```python
from build123d import *

# Parameters (mm, degrees)
BOSS_EXTRUDE1_DEPTH = 0.8
BOSS_EXTRUDE2_DEPTH = 1
BOSS_EXTRUDE3_START = 1
BOSS_EXTRUDE3_DEPTH = 1
CUT_EXTRUDE1_DEPTH  = 0.5
SKETCH5_W           = 18.969303985
SKETCH5_H           = 16.990491699
CUT_EXTRUDE2_DEPTH  = 4


with BuildPart() as part:
    # Sketch1 → Boss-Extrude1 (new body)
    with BuildSketch(Plane(origin=(0, 0, 0), x_dir=(1, 0, 0), z_dir=(0, 1, 0))):
        with BuildLine():
            Line((-5, 7.5), (-5, 5.590169944))
            ThreePointArc((-5, 5.590169944), (-6.846531969, 3.061862178), (-7.5, 0))
            Line((-7.5, 0), (-7.5, -7.5))
            Line((-7.5, -7.5), (7.5, -7.5))
            Line((7.5, -7.5), (7.5, 0))
            ThreePointArc((7.5, 0), (6.846531969, 3.061862178), (5, 5.590169944))
            Line((5, 5.590169944), (5, 7.5))
            Line((5, 7.5), (3, 7.5))
            Line((3, 7.5), (3, 5.5))
            Line((3, 5.5), (3, 5.123475383))
            ThreePointArc((3, 5.123475383), (3.101282966, 4.684946373), (3.384615385, 4.335248401))
            ThreePointArc((3.384615385, 4.335248401), (0, -5.5), (-3.384615385, 4.335248401))
            ThreePointArc((-3.384615385, 4.335248401), (-3.101282966, 4.684946373), (-3, 5.123475383))
            Line((-3, 5.123475383), (-3, 5.5))
            Line((-3, 5.5), (-3, 7.5))
            Line((-3, 7.5), (-5, 7.5))
        make_face()
    extrude(amount=BOSS_EXTRUDE1_DEPTH)

    # Sketch2 → Boss-Extrude2 (add)
    with BuildSketch(Plane(origin=(0, 0.8, 0), x_dir=(1, 0, 0), z_dir=(0, 1, 0))):
        with BuildLine():
            Line((5, 5.590169944), (5, 7.5))
            Line((5, 7.5), (3, 7.5))
            Line((3, 7.5), (-3, 7.5))
            Line((-3, 7.5), (-5, 7.5))
            Line((-5, 7.5), (-5, 5.590169944))
            ThreePointArc((-5, 5.590169944), (-6.846531969, 3.061862178), (-7.5, 0))
            Line((-7.5, 0), (-7.5, -7.5))
            Line((-7.5, -7.5), (7.5, -7.5))
            Line((7.5, -7.5), (7.5, 0))
            ThreePointArc((7.5, 0), (6.846531969, 3.061862178), (5, 5.590169944))
        make_face()
    extrude(amount=BOSS_EXTRUDE2_DEPTH)

    # Sketch3 → Boss-Extrude3 (add)
    with BuildSketch(Plane.XZ.offset(BOSS_EXTRUDE3_START)):
        with BuildLine():
            Line((-3, -7.5), (-5, -7.5))
            Line((-5, -7.5), (-5, -5.590169944))
            ThreePointArc((-5, -5.590169944), (-6.846531969, -3.061862178), (-7.5, 0))
            Line((-7.5, 0), (-7.5, 7.5))
            Line((-7.5, 7.5), (7.5, 7.5))
            Line((7.5, 7.5), (7.5, 0))
            ThreePointArc((7.5, 0), (6.846531969, -3.061862178), (5, -5.590169944))
            Line((5, -5.590169944), (5, -7.5))
            Line((5, -7.5), (3, -7.5))
            Line((3, -7.5), (-3, -7.5))
        make_face()
    extrude(amount=-BOSS_EXTRUDE3_DEPTH)

    # Sketch4 → Cut-Extrude1 (cut)
    with BuildSketch(Plane(origin=(0, 0, -7.5), x_dir=(-1, 0, 0), z_dir=(0, 0, -1))):
        Polygon((-5, 0.55), (-0.15, 0.55), (-0.15, 1.8), (0.15, 1.8), (0.15, 0.55), (5, 0.55), (5, 0.25), (0.15, 0.25), (0.15, -1), (-0.15, -1), (-0.15, 0.25), (-5, 0.25), align=None)
    extrude(amount=-CUT_EXTRUDE1_DEPTH, mode=Mode.SUBTRACT)

    # Sketch5 → Cut-Extrude2 (cut)
    with BuildSketch(Plane(origin=(0, 0.4, 0), x_dir=(-1, 0, 0), z_dir=(0, -1, 0))):
        with Locations((0.318429563, 0.045489938)):
            Rectangle(SKETCH5_W, SKETCH5_H)
    extrude(amount=CUT_EXTRUDE2_DEPTH, mode=Mode.SUBTRACT)


solid = part.part
```
Can you work these out from the model? Positions are in its coordinate system, mm. A direction names the side the tool comes from. Give positions to 0.01 mm unless a question says otherwise; leave off trailing zeros. Loops run counter-clockwise (first coordinate to the right, second up) from the corner with the lowest first, then second, coordinate; pieces in that order, holes last. Notation, with made-up numbers: M -19,14.25 L 38,14.25 A25 cw 38,39.25 Z; hole C 14.25,6 d8. An arc over 180 degrees is marked long. Use one line per item in the form item = value. Start each with the question number.
(1) Thinking about a two-plate mould opening in Z: for faces 4 (the cylindrical face through (0.191, 0.597, 5.497)), 5 (the flat face through (-7.5, 1, 4)), 6 (the flat face through (-3, 1, -7.5)), which applies, released by +Z, released by -Z, zero draft, split by the parting line, or undercut?
(2) On a 3-axis mill with a long thin cutter (end or side, diameter ignored), from which of +Z, -Z, +X, -X, +Y, -Y can I reach the whole of each face in a straight line? I mean faces 1 (the flat face through (5, 1, -7)), 2 (the flat face through (0, 0.8, -1)), 3 (the flat face through (-5, 1, -7)). Say none if no direction works.
(3) Please list where these lines run through material, in increasing order: line 1 (X direction, y = 0.7, z = 0); line 2 (X direction, y = 0.5, z = -6); line 3 (Z direction, x = 0, y = 1.4).
(4) I want a section at C-C, the plane x = -2.25. Write out the boundary of the cut face in (y, z).
(5) I want a section at D-D, the plane z = 3.5. Write out the boundary of the cut face in (x, y), and give its area (3 significant figures).
(6) I want a section at B-B, the plane z = 2. Write out the boundary of the cut face in (x, y), and give its area (3 significant figures).
(7) I'm going to push flat-ended pins straight in: P1, Ø5.5, axis at x = 2, z = -1.5, coming from the -Y side; P2, Ø0.7, axis at y = 1.5, z = -7, coming from the +X side. Where does each tip first touch, or does it pass through?
(8) I want a section at A-A, the plane y = 1.5. Write out the boundary of the cut face in (x, z), and give its area (3 significant figures).
Worked out:
q1.face_4 = undercut
q1.face_5 = zero draft
q1.face_6 = released by -Z
q2.face_1 = -Z, +X, +Y, -Y
q2.face_2 = -Y
q2.face_3 = -Z, -X, +Y, -Y
q3.line_1 = -7.5 to -5.5, 5.5 to 7.5
q3.line_2 = -5 to -3, 3 to 5
q3.line_3 = -7 to 7.5
q4.outline = M 0.4,5.02 L 0.8,5.02 L 0.8,-7.5 L 1.8,-7.5 L 1.8,7.5 L 0.4,7.5 Z
q5.outline = M -7.5,0.4 L -4.24,0.4 L -4.24,0.8 L 4.24,0.8 L 4.24,0.4 L 7.5,0.4 L 7.5,1.8 L -7.5,1.8 Z
q5.area = 17.6 mm²
q6.outline = M -7.5,0.4 L -5.12,0.4 L -5.12,0.8 L 5.12,0.8 L 5.12,0.4 L 7.5,0.4 L 7.5,1.8 L -7.5,1.8 Z
q6.area = 16.9 mm²
q7.P1 = 0.8
q7.P2 = 5
q8.outline = M -7.5,0 A7.5 ccw -5,-5.59 L -5,-7.5 L -0.15,-7.5 L -0.15,-7 L 0.15,-7 L 0.15,-7.5 L 5,-7.5 L 5,-5.59 A7.5 ccw 7.5,0 L 7.5,7.5 L -7.5,7.5 Z
q8.area = 207 mm²
